```python
from build123d import *

# Parameters (mm, degrees)
F1_W     = 12
F1_H     = 2
F4_DEPTH = 2
F5_R     = 2.5
F6_DEPTH = 2
F7_R     = 5.99999
F8_R     = 5.99999


# Not quite as in the source:
# - a fillet or chamfer is up to 0.001 mm smaller than in the source, because OpenCascade refuses the exact size


with BuildPart() as f2:
    # F2: sweep along a path in F0
    with BuildLine(Plane.YZ) as f2_path:
        Line((0, 0), (16.9722436227, 0))
        ThreePointArc((16.9722436227, 0), (19.8700851096, 0.4290797351), (22.5192455849, 1.6794970566))
        Line((22.5192455849, 1.6794970566), (32.4807544151, 8.3205029434))
        ThreePointArc((32.4807544151, 8.3205029434), (35.1299148904, 9.5709202649), (38.0277563773, 10))
        Line((38.0277563773, 10), (92, 10))
    # F1 (on Front) → F2 (sweep)
    with BuildSketch(Plane.XZ):
        with Locations((0, 1)):
            Rectangle(F1_W, F1_H)
    sweep(path=f2_path.line)

    # F3 (on Top) → F4 (cut, through all)
    with BuildSketch(Plane.XY):
        with BuildLine():
            Line((2, 4.5), (2, 7.5))
            ThreePointArc((2, 7.5), (0, 8.5), (-2, 7.5))
            Line((-2, 7.5), (-2, 4.5))
            ThreePointArc((-2, 4.5), (0, 3.5), (2, 4.5))
        make_face()
    extrude(amount=F4_DEPTH, mode=Mode.SUBTRACT)

    # F5 (on face) → F6 (cut, through all)
    with BuildSketch(Plane.XY.offset(12)):
        with Locations((0, 86)):
            Circle(F5_R)
    extrude(amount=-F6_DEPTH, mode=Mode.SUBTRACT)

    # F7 (radius 6 in the source; OpenCascade refuses exactly that, so slightly less here)
    f7_edges = [f2.edges().sort_by_distance(p)[0] for p in [
        (6, 0, 1),
        (-6, 0, 1),
    ]]
    fillet(f7_edges, radius=F7_R)

    # F8 (radius 6 in the source; OpenCascade refuses exactly that, so slightly less here)
    f8_edges = [f2.edges().sort_by_distance(p)[0] for p in [
        (-6, 92, 11),
        (6, 92, 11),
    ]]
    fillet(f8_edges, radius=F8_R)


solid = f2.part
```
Design review of the part built by this model. Coordinates are the model's own, in mm. A direction names the side the tool comes from. Round coordinates to 2 decimals unless told otherwise and drop trailing zeros. Write each loop counter-clockwise with the first axis right and the second up, starting at its lowest first coordinate (ties: lowest second). Pieces come first, ordered by that corner, then holes.
Item 1: We need section A-A on y = 49. Write out the cut boundary in (x, z).
Item 2: The part is to be moulded in two halves that separate along X. For faces 5 (the flat face through (-6, 46, 11)), 6 (the cylindrical face through (0.08, 35.09, 9.56)), 7 (the cylindrical face through (4.196, 1.711, 1.014)), 8 (the cylindrical face through (0, 3.5, 1)), say which applies: +X half, -X half, draft (parallel to the pull), parting line (faces both ways), or undercut.
Item 3: We need section C-C on z = 5.25. Write out the cut boundary in (x, y) (3 decimals).
Item 4: For probe 1 along Z at (x, y) = (2.25, 71); probe 2 along Z at (x, y) = (2.25, 12.5); probe 3 along Y at (x, z) = (0, 10.75), list the stretches that pass through material, from the lowest coordinate up.
Item 5: Clearance check with flat-ended pins moving along their axes: pin 1 Ø4 at (x, y) = (1, 81.5) entering from -Z; pin 2 Ø6 at (x, z) = (1, 2.5) entering from +Y; pin 3 Ø3 at (y, z) = (48.5, 8) entering from -X; pin 4 Ø4 at (x, z) = (-2.5, 2.5) entering from +Y. State where each tip first meets the part, or that it passes through.
Item 6: We need section B-B on x = 5.25. Write out the cut boundary in (y, z).
Item 7: For faces 1 (the flat face through (0, 9, 2)), 2 (the flat face through (0, 65, 10)), 3 (the flat face through (2, 6, 1)), 4 (the flat face through (0, 9, 0)), list the 3-axis set-ups (+Z, -Z, +X, -X, +Y, -Y) from which the entire face can be reached by the end or side of a thin tool; tool diameter is ignored.
Returned:
1. outline: (-6, 10) - (6, 10) - (6, 12) - (-6, 12) - close
2. face 5: -X half
2. face 6: draft
2. face 7: +X half
2. face 8: undercut
3. outline: (-6, 24.269) - (6, 24.269) - (6, 27.875) - (-6, 27.875) - close
4. probe 1: z = 10 to 12
4. probe 2: z = 0 to 2
4. probe 3: y = 32.7 to 83.5, 88.5 to 92
5. pin 1: stops at z = 10
5. pin 2: stops at y = 28.25
5. pin 3: passes through
5. pin 4: stops at y = 26.75
6. outline: (3.1, 0) - (16.97, 0) arc R10 ccw to (22.52, 1.68) - (32.48, 8.32) arc R10 cw to (38.03, 10) - (88.9, 10) - (88.9, 12) - (38.03, 12) arc R12 ccw to (31.37, 9.98) - (21.41, 3.34) arc R8 cw to (16.97, 2) - (3.1, 2) - close
7. face 1: +Z, +X, -X, -Y
7. face 2: -Z, +X, -X, +Y
7. face 3: +Z, -Z
7. face 4: -Z, +X, -X, +Y, -Y
